```python
from build123d import *

# Parameters (mm, degrees)
F0_R     = 3.5
F1_DEPTH = 15
F3_DEPTH = 5
F4_SIZE  = 2


with BuildPart() as f1:
    # F0 (on Top) → F1 (new body)
    with BuildSketch(Plane.XY):
        with BuildLine():
            Line((-250, 30), (-250, -30))
            Line((-250, -30), (-200, -30))
            Line((-200, -30), (-200, -10))
            ThreePointArc((-200, -10), (-175, 15), (-150, -10))
            Line((-150, -10), (-150, -30))
            Line((-150, -30), (-130, -30))
            Line((-130, -30), (-130, -10))
            ThreePointArc((-130, -10), (-105, 15), (-80, -10))
            Line((-80, -10), (-80, -30))
            Line((-80, -30), (-60, -30))
            Line((-60, -30), (-60, -10))
            ThreePointArc((-60, -10), (-35, 15), (-10, -10))
            Line((-10, -10), (-10, -30))
            Line((-10, -30), (10, -30))
            Line((10, -30), (10, -10))
            ThreePointArc((10, -10), (35, 15), (60, -10))
            Line((60, -10), (60, -30))
            Line((60, -30), (80, -30))
            Line((80, -30), (80, -10))
            ThreePointArc((80, -10), (105, 15), (130, -10))
            Line((130, -10), (130, -30))
            Line((130, -30), (150, -30))
            Line((150, -30), (150, -10))
            ThreePointArc((150, -10), (175, 15), (200, -10))
            Line((200, -10), (200, -30))
            Line((200, -30), (250, -30))
            Line((250, -30), (250, 30))
            Line((250, 30), (-250, 30))
        make_face()
        with Locations((-225, 0)):
            Circle(F0_R, mode=Mode.SUBTRACT)
        with Locations((225, 0)):
            Circle(F0_R, mode=Mode.SUBTRACT)
    extrude(amount=F1_DEPTH)

    # F2 (on face) → F3 (join)
    with BuildSketch(Plane(origin=(0, 0, 0), x_dir=(1, 0, 0), z_dir=(0, 0, -1))):
        with BuildLine():
            Line((-200, 20), (-200, 10))
            ThreePointArc((-200, 10), (-175, -15), (-150, 10))
            Line((-150, 10), (-150, 20))
            Line((-150, 20), (-156, 10))
            ThreePointArc((-156, 10), (-175, -9), (-194, 10))
            Line((-194, 10), (-200, 20))
        make_face()
        with BuildLine():
            ThreePointArc((-86, 10), (-105, -9), (-124, 10))
            Line((-124, 10), (-130, 20))
            Line((-130, 20), (-130, 10))
            ThreePointArc((-130, 10), (-105, -15), (-80, 10))
            Line((-80, 10), (-80, 20))
            Line((-80, 20), (-86, 10))
        make_face()
        with BuildLine():
            ThreePointArc((-16, 10), (-35, -9), (-54, 10))
            Line((-54, 10), (-60, 20))
            Line((-60, 20), (-60, 10))
            ThreePointArc((-60, 10), (-35, -15), (-10, 10))
            Line((-10, 10), (-10, 20))
            Line((-10, 20), (-16, 10))
        make_face()
        with BuildLine():
            ThreePointArc((54, 10), (35, -9), (16, 10))
            Line((16, 10), (10, 20))
            Line((10, 20), (10, 10))
            ThreePointArc((10, 10), (35, -15), (60, 10))
            Line((60, 10), (60, 20))
            Line((60, 20), (54, 10))
        make_face()
        with BuildLine():
            ThreePointArc((124, 10), (105, -9), (86, 10))
            Line((86, 10), (80, 20))
            Line((80, 20), (80, 10))
            ThreePointArc((80, 10), (105, -15), (130, 10))
            Line((130, 10), (130, 20))
            Line((130, 20), (124, 10))
        make_face()
        with BuildLine():
            ThreePointArc((194, 10), (175, -9), (156, 10))
            Line((156, 10), (150, 20))
            Line((150, 20), (150, 10))
            ThreePointArc((150, 10), (175, -15), (200, 10))
            Line((200, 10), (200, 20))
            Line((200, 20), (194, 10))
        make_face()
    extrude(amount=-F3_DEPTH)

    # F4
    f4_edges = [f1.edges().sort_by_distance(p)[0] for p in [
        (-197, -15, 5),
        (-197, -15, 0),
        (-57, -15, 0),
        (-57, -15, 5),
        (-127, -15, 5),
        (-127, -15, 0),
        (-153, -15, 5),
        (-153, -15, 0),
        (-83, -15, 5),
        (-83, -15, 0),
        (-13, -15, 0),
        (-13, -15, 5),
        (57, -15, 5),
        (57, -15, 0),
        (127, -15, 5),
        (127, -15, 0),
        (197, -15, 5),
        (197, -15, 0),
        (13, -15, 5),
        (13, -15, 0),
        (83, -15, 5),
        (83, -15, 0),
        (153, -15, 5),
        (153, -15, 0),
    ]]
    chamfer(f4_edges, length=F4_SIZE)


solid = f1.part
```
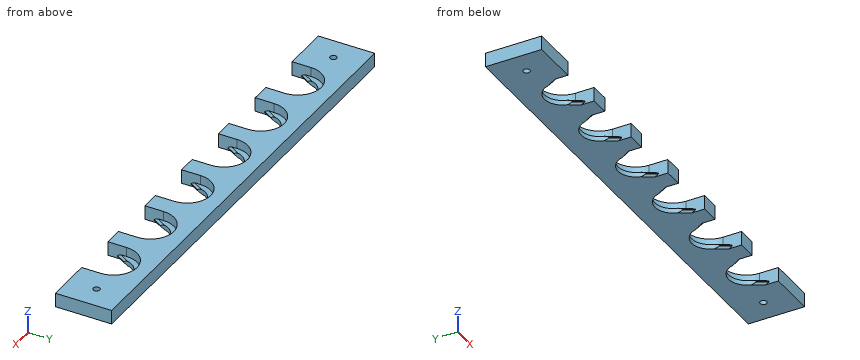
Input: part model. Units: mm. Frame: model coordinates. Coordinates: 2 decimals unless noted, no trailing zeros. Write each loop counter-clockwise with the first axis right and the second up, starting at its lowest first coordinate (ties: lowest second). Pieces come first, ordered by that corner, then holes.
1) Material intervals for line 1 along Y through (x, z) = (-225, 7.5); line 2 along Z through (x, y) = (-199.5, -7); line 3 along Y through (x, z) = (-227, 11.5), sorted ascending.
2) Section C-C on x = -175.5. Output: boundary loops of the cut face in (y, z) (3 decimals).
3) Section A-A on z = 7.75. State how many separate pieces and enclosed holes the cut face has, and give its area (3 significant figures).
4) Pin query (flat end, axial travel): pin 1 Ø15.5 at (x, y) = (-165.5, -3) entering from +Z; pin 2 Ø25 at (x, y) = (-94, 5.5) entering from +Z; pin 3 Ø6.5 at (x, y) = (-225, 0) entering from +Z. Return the tip coordinate at first contact, or that it passes through.
5) Section B-B on x = -105. Output: boundary loops of the cut face in (y, z).
Check result:
1. line 1: y = -30 to -3.5, 3.5 to 30
1. line 2: z = 0 to 5
1. line 3: y = -30 to -2.87, 2.87 to 30
2. outline: (8.993, 0) - (30, 0) - (30, 15) - (14.995, 15) - (14.995, 5) - (8.993, 5) - close
3. separate pieces: 1
3. enclosed holes: 2
3. area: 18,000 mm2
4. pin 1: stops at z = 5
4. pin 2: stops at z = 15
4. pin 3: passes through
5. outline: (9, 0) - (30, 0) - (30, 15) - (15, 15) - (15, 5) - (9, 5) - close
